Verification items for the finished model (mm, model axes). Face numbers are marked on the shaded views. A direction names the side the tool comes from. Give positions to 0.01 mm unless a question says otherwise; leave off trailing zeros. Loops run counter-clockwise (first coordinate to the right, second up) from the corner with the lowest first, then second, coordinate; pieces in that order, holes last. Notation, with made-up numbers: (-11.75, 12) - (2.25, 12) arc R13 ccw to (2.25, 34) - close; hole circle Ø7 at (83.5, 17). An arc over 180 degrees is marked (long way). Use one line per item in the form item = value.
```python
from build123d import *

# Parameters (mm, degrees)
ESBO_O1_R                = 18.5
ESBO_O1_R_2              = 12
RESSALTO_EXTRUS_O1_DEPTH = 4
RESSALTO_EXTRUS_O2_DEPTH = 27
FILETE1_R                = 0.5
ESBO_O3_W                = 39
ESBO_O3_H                = 7
RESSALTO_EXTRUS_O3_DEPTH = 75
ESBO_O4_R                = 1.55
CORTE_EXTRUS_O1_DEPTH    = 7
ESBO_O5_R                = 3.6
CORTE_EXTRUS_O2_DEPTH    = 3.5
ESBO_O6_R                = 1.55
CORTE_EXTRUS_O4_DEPTH    = 4


with BuildPart() as part:
    # Esboço1 → Ressalto-extrusão1 (new body)
    with BuildSketch(Plane(origin=(0, 0, 0), x_dir=(0, 0, -1), z_dir=(1, 0, 0))):
        Circle(ESBO_O1_R)
        Circle(ESBO_O1_R_2, mode=Mode.SUBTRACT)
    extrude(amount=RESSALTO_EXTRUS_O1_DEPTH)

    # Esboço2 → Ressalto-extrusão2 (add)
    with BuildSketch(Plane.ZY):
        with BuildLine():
            Line((-19.5, 0), (-19.5, -21))
            Line((-19.5, -21), (19.5, -21))
            Line((19.5, -21), (19.5, 0))
            Line((19.5, 0), (18.5, 0))
            ThreePointArc((18.5, 0), (0, -18.5), (-18.5, 0))
            Line((-18.5, 0), (-19.5, 0))
        make_face()
    extrude(amount=-RESSALTO_EXTRUS_O2_DEPTH)

    # Filete1
    filete1_edges = [part.edges().sort_by_distance(p)[0] for p in [
        (2, 0, 18.5),
        (2, 0, -18.5),
    ]]
    fillet(filete1_edges, radius=FILETE1_R)

    # Esboço3 → Ressalto-extrusão3 (add)
    with BuildSketch(Plane.ZY):
        with Locations((0, -24.5)):
            Rectangle(ESBO_O3_W, ESBO_O3_H)
    extrude(amount=-RESSALTO_EXTRUS_O3_DEPTH)

    # Esboço4 → Corte-extrusão1 (cut)
    with BuildSketch(Plane(origin=(0, -21, 0), x_dir=(1, 0, 0), z_dir=(0, 1, 0))):
        with Locations(Location((33, 13.5, 0), (0, 0, 270))):
            Circle(ESBO_O4_R)
        with Locations(Location((69, 13.5, 0), (0, 0, 270))):
            Circle(ESBO_O4_R)
        with Locations(Location((33, -13.5, 0), (0, 0, 270))):
            Circle(ESBO_O4_R)
        with Locations(Location((69, -13.5, 0), (0, 0, 270))):
            Circle(ESBO_O4_R)
    extrude(amount=-CORTE_EXTRUS_O1_DEPTH, mode=Mode.SUBTRACT)

    # Esboço5 → Corte-extrusão2 (cut)
    with BuildSketch(Plane(origin=(0, -21, 0), x_dir=(1, 0, 0), z_dir=(0, 1, 0))):
        with Locations(Location((33, 13.5, 0), (0, 0, 270))):
            Circle(ESBO_O5_R)
        with Locations(Location((69, 13.5, 0), (0, 0, 270))):
            Circle(ESBO_O5_R)
        with Locations(Location((69, -13.5, 0), (0, 0, 270))):
            Circle(ESBO_O5_R)
        with Locations(Location((33, -13.5, 0), (0, 0, 270))):
            Circle(ESBO_O5_R)
    extrude(amount=-CORTE_EXTRUS_O2_DEPTH, mode=Mode.SUBTRACT)

    # Esboço6 → Corte-extrusão4 (cut)
    with BuildSketch(Plane.ZY):
        with Locations(Location((9.899494937, 9.899494937, 0), (0, 0, 180))):
            Circle(ESBO_O6_R)
        with Locations(Location((9.899494937, -9.899494937, 0), (0, 0, 180))):
            Circle(ESBO_O6_R)
        with Locations(Location((-9.899494937, -9.899494937, 0), (0, 0, 180))):
            Circle(ESBO_O6_R)
        with Locations(Location((-9.899494937, 9.899494937, 0), (0, 0, 180))):
            Circle(ESBO_O6_R)
    extrude(amount=-CORTE_EXTRUS_O4_DEPTH, mode=Mode.SUBTRACT)


solid = part.part
```
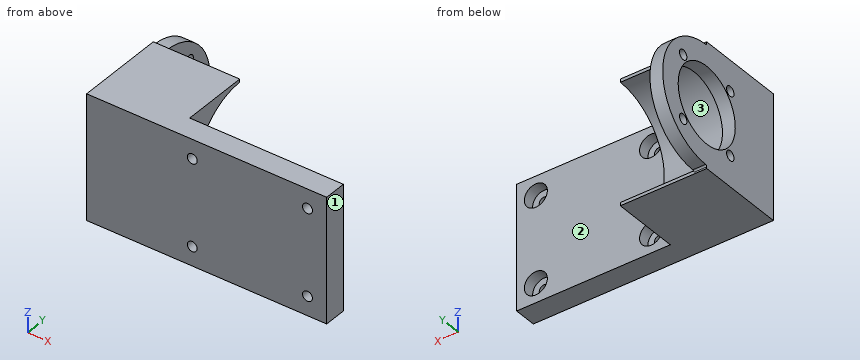
1. Depth check by flat-ended pin: pin 1 Ø1.9 at (x, z) = (69, -13.5) entering from +Y; pin 2 Ø0.5 at (x, z) = (13, -19) entering from +Y; pin 3 Ø12 at (x, z) = (64.5, -7.5) entering from +Y; pin 4 Ø2 at (x, z) = (70, 12) entering from +Y. Enter the tip coordinate at first touch or a pass-through.
Result set:
pin_1 = through
pin_2 = 0
pin_3 = -21
pin_4 = -24.5
2. Section check D-D, the plane z = -13. Record the cut outline in (x, y), then the cut area to 3 significant figures.
Result set:
outline = (0, -28) - (31.53, -28) - (31.53, -24.5) - (29.43, -24.5) - (29.43, -21) - (27, -21) - (27, -13.16) - (4, -13.16) - (4, 13.16) - (0, 13.16) - close; (34.47, -28) - (67.53, -28) - (67.53, -24.5) - (65.43, -24.5) - (65.43, -21) - (36.57, -21) - (36.57, -24.5) - (34.47, -24.5) - close; (70.47, -28) - (75, -28) - (75, -21) - (72.57, -21) - (72.57, -24.5) - (70.47, -24.5) - close
area = 771 mm²
3. Scan lines: probe 1 along X at (y, z) = (-25.75, 13.5); probe 2 along Z at (x, y) = (69, -27.05); probe 3 along X at (y, z) = (-18.5, -11.5). Record each from-to range of solid material in increasing order.
Result set:
probe_1 = 0 to 31.45, 34.55 to 67.45, 70.55 to 75
probe_2 = -19.5 to -15.05, -11.95 to 11.95, 15.05 to 19.5
probe_3 = 0 to 27
4. Section check B-B, the plane x = 33. Record the cut outline in (y, z).
Result set:
outline = (-28, -19.5) - (-21, -19.5) - (-21, -17.1) - (-24.5, -17.1) - (-24.5, -15.05) - (-28, -15.05) - close; (-28, -11.95) - (-24.5, -11.95) - (-24.5, -9.9) - (-21, -9.9) - (-21, 9.9) - (-24.5, 9.9) - (-24.5, 11.95) - (-28, 11.95) - close; (-28, 15.05) - (-24.5, 15.05) - (-24.5, 17.1) - (-21, 17.1) - (-21, 19.5) - (-28, 19.5) - close
5. Tool access check on the marked faces 1, 2 and 3. Record the directions out of +Z, -Z, +X, -X, +Y, -Y that give a thin tool (end or side, any length) a straight path to the whole face; none if there is none.
Result set:
face_1 = +Z, -Z, +X, +Y, -Y
face_2 = +Z, -Z, +X, +Y
face_3 = +X, +Y
6. Section check A-A, the plane z = 0. Record the cut outline in (x, y), then the cut area to 4 significant figures.
Result set:
outline = (0, -28) - (75, -28) - (75, -21) - (27, -21) - (27, -18.5) - (4, -18.5) - (4, -12) - (0, -12) - close; (0, 12) - (4, 12) - (4, 18.5) - (0, 18.5) - close
area = 644.5 mm²
7. Section check C-C, the plane y = 3. Record the cut outline in (x, z).
Result set:
outline = (0, -18.26) - (4, -18.26) - (4, -11.62) - (0, -11.62) - close; (0, 11.62) - (4, 11.62) - (4, 18.26) - (0, 18.26) - close
